Geometry check sheet. Reference: the model listing, model coordinates, mm. A direction names the side the tool comes from. Coordinates: 2 decimals unless noted, no trailing zeros. Order: outer loops, then holes, each group sorted by start corner. A loop starts at its lowest first (then second) coordinate and runs counter-clockwise, first axis right, second up. Notation, with made-up numbers: (-3, 83) - (18, 83) arc R34 cw to (18, 117) - close; hole circle Ø7 at (-28, 26.5). An arc over 180 degrees is marked (long way). Return JSON: item names as keys, results as strings. Group by question number.
Item 1: Gauge pin test, flat ends, axial feed: pin 1 (8 mm diameter, centred on x = 18, y = 85, fed in from -Z); pin 2 (16 mm diameter, centred on x = -6.5, z = 3.5, fed in from +Y); pin 3 (17.5 mm diameter, centred on y = 62, z = 7.5, fed in from -X). Record the tip position at first contact, or that the pin passes through.
Item 2: Section check B-B on x = -25. Enter the section's corners in (y, z), then the cut area to 3 significant figures.
Item 3: Tool access check on faces 5 (the flat face through (-15, 53, -9.5)), 6 (the flat face through (-9.5, 53, -15)), 7 (the cylindrical face through (-13.887, 106.479, -10.648)). Record the directions out of +Z, -Z, +X, -X, +Y, -Y that give a thin tool (end or side, any length) a straight path to the whole face; none if there is none.
Item 4: Section check D-D on z = 3. Enter the section's corners in (x, y).
Item 5: Section check C-C on z = -2.5. Enter the section's corners in (x, y).
Item 6: Section check A-A on y = 61. Enter the section's corners in (x, z), then the cut area to 3 significant figures.
Item 7: Draft check along Y on faces 1 (the flat face through (16.2, 8, -0.1)), 2 (the flat face through (-9.5, 53, 15)), 3 (the flat face through (0, 0, 0)), 4 (the flat face through (0, 106, -22)). Enter one of: pulls with the +Y half, pulls with the -Y half, needs draft (parallel to the pull), parting line crosses it, or undercut.
Item 8: Scan lines: probe 1 along Z at (x, y) = (-25, 105.9); probe 2 along Z at (x, y) = (-16, 49); probe 3 along Y at (x, z) = (5, -15.5). Record each from-to range of solid material in increasing order.
Autodesk Inventor part; units mm, degrees
ref_plane "YZ Plane" through (0, 0, 0) normal (1, 0, 0) x (0, 1, 0)
ref_plane "XZ Plane" through (0, 0, 0) normal (0, 1, 0) x (-1, 0, 0)
ref_plane "XY Plane" through (0, 0, 0) normal (0, 0, 1) x (1, 0, 0)
sketch "Sketch1" plane through (0, 0, 0) normal (0, 1, 0) x (-1, 0, 0)
  line L0 (17.5, 17.5) -> (-17.5, 17.5)
  line L1 (-17.5, 17.5) -> (-17.5, -17.5)
  line L2 (-17.5, -17.5) -> (17.5, -17.5)
  line L3 (17.5, -17.5) -> (17.5, 17.5)
  line L4 (17.5, 17.5) -> (-17.5, -17.5) construction
  line L5 (-17.5, 17.5) -> (17.5, -17.5) construction
  circle A0 centre (0, 0) radius 16
  dimension "d0" = 35
  dimension "d1" = 35
  dimension "d2" = 32
extrude "Extrusion1" add sketch "Sketch1" along normal blind 105
sketch "Sketch2" plane through (17.5, 0, 17.5) normal (1, 0, 0) x (0, 0, -1)
  line L0 (27, 8) -> (8, 8)
  line L1 (8, 8) -> (8, 97)
  line L2 (8, 97) -> (27, 97)
  line L3 (27, 97) -> (27, 8)
  line L4 (0, 0) -> (35, 0)
  line L5 (0, 0) -> (0, 105)
  line L6 (35, 0) -> (35, 105)
  line L7 (0, 105) -> (35, 105)
  point P0 (17.5, 0)
  dimension "d5" = 8
  dimension "d6" = 8
  dimension "d7" = 8
  dimension "d8" = 8
extrude "Extrusion2" cut sketch "Sketch2" against normal through all contours L0 L1 L2 L3
sketch "Sketch3" plane through (17.5, 0, -17.5) normal (0, 0, -1) x (-1, 0, 0)
  line L0 (8, 97) -> (27, 97)
  line L1 (27, 97) -> (27, 8)
  line L2 (27, 8) -> (8, 8)
  line L3 (8, 8) -> (8, 97)
  line L4 (0, 0) -> (0, 105)
  line L5 (35, 0) -> (35, 105)
  line L6 (0, 105) -> (35, 105)
  line L7 (0, 0) -> (35, 0)
  point P0 (17.5, 0)
  dimension "d11" = 8
  dimension "d12" = 8
  dimension "d13" = 8
  dimension "d14" = 8
extrude "Extrusion3" cut sketch "Sketch3" against normal through all contours L0 L1 L2 L3
sketch "Sketch4" plane through (0, 0, 0) normal (0, -1, 0) x (1, 0, 0)
  line L0 (17.5, 17.5) -> (17.5, -17.5)
  line L1 (-17.5, 17.5) -> (17.5, 17.5)
  line L2 (17.5, 17.5) -> (17.5, -17.5)
  line L3 (17.5, -17.5) -> (-17.5, -17.5)
  line L4 (-17.5, -17.5) -> (-17.5, 17.5)
  line L5 (-17.5, 17.5) -> (17.5, -17.5) construction
  line L6 (17.5, 17.5) -> (-17.5, -17.5) construction
  point P0 (0, 0)
extrude "Extrusion4" add sketch "Sketch4" along normal blind 3
sketch "Sketch5" plane through (0, 105, 0) normal (0, 1, 0) x (1, 0, 0)
  line L0 (30, 22) -> (-30, 22)
  line L1 (-30, 22) -> (-30, -22)
  line L2 (-30, -22) -> (30, -22)
  line L3 (30, -22) -> (30, 22)
  line L4 (30, 22) -> (-30, -22) construction
  line L5 (-30, 22) -> (30, -22) construction
  circle A0 centre (0, 0) radius 17.5
  circle A1 centre (25, -17.5) radius 2.7
  circle A2 centre (25, 17.5) radius 2.7
  circle A3 centre (-25, 17.5) radius 2.7
  circle A4 centre (-25, -17.5) radius 2.7
  dimension "d19" = 60
  dimension "d20" = 44
  dimension "d21" = 35
  dimension "d22" = 5.4
  dimension "d23" = 4.5
  dimension "d24" = 5
  dimension "d25" = 5.4
  dimension "d26" = 4.5
  dimension "d27" = 5
  dimension "d28" = 4.5
  dimension "d29" = 5
  dimension "d30" = 5.4
  dimension "d31" = 5.4
  dimension "d32" = 4.5
  dimension "d33" = 5
extrude "Extrusion5" add sketch "Sketch5" along normal blind 3
equation "\"d0\" = d1"
equation "\"d6\" = d5"
equation "\"d7\" = d6"
equation "\"d8\" = d5"
equation "\"d12\" = d11"
equation "\"d13\" = d11"
equation "\"d14\" = d11"
equation "\"d25\" = d22"
equation "\"d26\" = d23"
equation "\"d27\" = d24"
equation "\"d28\" = d32"
equation "\"d29\" = d24"
equation "\"d30\" = d22"
equation "\"d31\" = d22"
equation "\"d32\" = d23"
equation "\"d33\" = d24"
properties part number "port tube v01"
Computed:
{
 "1": {"pin 1": "stops at z = -17.5", "pin 2": "stops at y = 0", "pin 3": "stops at x = -17.5"},
 "2": {"outline": "(105, -22) - (108, -22) - (108, -20.2) - (105, -20.2) - close; (105, -14.8) - (108, -14.8) - (108, 14.8) - (105, 14.8) - close; (105, 20.2) - (108, 20.2) - (108, 22) - (105, 22) - close", "area": "99.6 mm²"},
 "3": {"face 5": "+X, -X", "face 6": "+Z, -Z", "face 7": "+Y"},
 "4": {"outline": "(-30, 105) - (-17.5, 105) - (-17.5, 97) - (-15.72, 97) - (-15.72, 105) - (-17.24, 105) - (-17.24, 108) - (-30, 108) - close; (-17.5, -3) - (17.5, -3) - (17.5, 8) - (15.72, 8) - (15.72, 0) - (-15.72, 0) - (-15.72, 8) - (-17.5, 8) - close; (15.72, 97) - (17.5, 97) - (17.5, 105) - (30, 105) - (30, 108) - (17.24, 108) - (17.24, 105) - (15.72, 105) - close"},
 "5": {"outline": "(-30, 105) - (-17.5, 105) - (-17.5, 97) - (-15.8, 97) - (-15.8, 105) - (-17.32, 105) - (-17.32, 108) - (-30, 108) - close; (-17.5, -3) - (17.5, -3) - (17.5, 8) - (15.8, 8) - (15.8, 0) - (-15.8, 0) - (-15.8, 8) - (-17.5, 8) - close; (15.8, 97) - (17.5, 97) - (17.5, 105) - (30, 105) - (30, 108) - (17.32, 108) - (17.32, 105) - (15.8, 105) - close"},
 "6": {"outline": "(-17.5, -17.5) - (-9.5, -17.5) - (-9.5, -12.87) arc R16 cw to (-12.87, -9.5) - (-17.5, -9.5) - close; (-17.5, 9.5) - (-12.87, 9.5) arc R16 cw to (-9.5, 12.87) - (-9.5, 17.5) - (-17.5, 17.5) - close; (9.5, -17.5) - (17.5, -17.5) - (17.5, -9.5) - (12.87, -9.5) arc R16 cw to (9.5, -12.87) - close; (9.5, 12.87) arc R16 cw to (12.87, 9.5) - (17.5, 9.5) - (17.5, 17.5) - (9.5, 17.5) - close", "area": "231 mm²"},
 "7": {"face 1": "undercut", "face 2": "undercut", "face 3": "pulls with the +Y half", "face 4": "needs draft"},
 "8": {"probe 1": "z = -22 to -20.2, -14.8 to 14.8, 20.2 to 22", "probe 2": "z = -17.5 to -9.5, 9.5 to 17.5", "probe 3": "y = -3 to 8, 97 to 105"}
}
